Can you work these out from the model? Positions are in its coordinate system, mm. A direction names the side the tool comes from. Give positions to 0.01 mm unless a question says otherwise; leave off trailing zeros. Loops run counter-clockwise (first coordinate to the right, second up) from the corner with the lowest first, then second, coordinate; pieces in that order, holes last. Notation, with made-up numbers: (2.25, 85) - (32.25, 85) arc R8 ccw to (32.25, 91) - close; hole circle Ø4 at (65.25, 3). An arc over 180 degrees is marked (long way). Answer as a JSON object with one key per item and string values. Group by question number.
Item 1: Suppose I cut it at A-A on x = 0. Write out the boundary of the cut face in (y, z), and give its area (3 significant figures).
Item 2: Which directions (+Z, -Z, +X, -X, +Y, -Y) give clear straight access to the entire face, cutting with the end or side of a thin tool? Please do faces 4 (the flat face through (6, 0, -32.871)), 5 (the flat face through (-10, -10, -42.871)), 6 (the flat face through (6, 0, 32.871)), 7 (the conical face through (-40.938, 12.892, -29.206)), 8 (the cylindrical face through (49.45, 2.18, -38.84)).
Item 3: Please list where these lines run through material, in increasing order: L1, parallel to X at y = 0.5, z = 20.5; L2, parallel to Y at x = 0, z = 35; L3, parallel to Y at x = 0, z = 12.
Item 4: Suppose I cut it at C-C on z = 13. Write out the boundary of the cut face in (x, y).
Item 5: Thinking about a two-plate mould opening in Y: for faces 1 (the flat face through (10, -10, 42.871)), 2 (the cylindrical face through (9.21, -41.47, -0.4)), 3 (the cylindrical face through (-10.316, 7.91, -37.941)), which applies, pulls with the +Y half, pulls with the -Y half, needs draft (parallel to the pull), parting line crosses it, or undercut?
Item 6: Will these pins go through, and if not, where does the flat tip stop? pin 1 (12 mm diameter, centred on y = -29.5, z = -17.5, fed in from -X); pin 2 (8 mm diameter, centred on y = 22.5, z = -8.5, fed in from +X); pin 3 (5 mm diameter, centred on y = 16, z = -13.5, fed in from -X).
from build123d import *

# Parameters (mm, degrees)
F2_R     = 5
F3_DEPTH = 1000
F2_R_2   = 13
F4_DEPTH = 10
F5_R     = 13
F5_R_2   = 5
F6_DEPTH = 10


with BuildPart() as f1:
    # F0 (on Front) → F1 (revolve)
    with BuildSketch(Plane.XZ):
        Polygon((0, 0), (0, 42.870745), (-49.496219, 42.870745), (-49.496219, 34.686334), (-42.481005, 28.84032), (-42.481005, 0), (-42.481005, -28.84032), (-49.496219, -34.686334), (-49.496219, -42.870745), (0, -42.870745), align=None)
    revolve(axis=Axis((0, 0, 21.435373), (0, 0, -1)))

    # F2 (on face) → F3 (cut)
    with BuildSketch(Plane.XY.offset(42.870745)):
        Circle(F2_R)
    extrude(amount=-F3_DEPTH, mode=Mode.SUBTRACT)

    # F2 (on face) → F4 (cut)
    with BuildSketch(Plane.XY.offset(42.870745)):
        Circle(F2_R_2)
        Circle(F2_R, mode=Mode.SUBTRACT)
    extrude(amount=-F4_DEPTH, mode=Mode.SUBTRACT)

    # F5 (on face) → F6 (cut)
    with BuildSketch(Plane(origin=(0, 0, -42.870745), x_dir=(1, 0, 0), z_dir=(0, 0, -1))):
        Circle(F5_R)
        Circle(F5_R_2, mode=Mode.SUBTRACT)
    extrude(amount=-F6_DEPTH, mode=Mode.SUBTRACT)


solid = f1.part
Worked out:
{
 "1": {"outline": "(-49.5, -42.87) - (-13, -42.87) - (-13, -32.87) - (-5, -32.87) - (-5, 32.87) - (-13, 32.87) - (-13, 42.87) - (-49.5, 42.87) - (-49.5, 34.69) - (-42.48, 28.84) - (-42.48, -28.84) - (-49.5, -34.69) - close; (5, -32.87) - (13, -32.87) - (13, -42.87) - (49.5, -42.87) - (49.5, -34.69) - (42.48, -28.84) - (42.48, 28.84) - (49.5, 34.69) - (49.5, 42.87) - (13, 42.87) - (13, 32.87) - (5, 32.87) - close", "area": "6,420 mm2"},
 "2": {"face 4": "-Z", "face 5": "-Z, +X, -X, +Y, -Y", "face 6": "+Z", "face 7": "none", "face 8": "+Z, -Z"},
 "3": {"L1": "x = -42.48 to -4.97, 4.97 to 42.48", "L2": "y = -49.5 to -13, 13 to 49.5", "L3": "y = -42.48 to -5, 5 to 42.48"},
 "4": {"outline": "circle Ø84.96 at (0, 0); hole circle Ø10 at (0, 0)"},
 "5": {"face 1": "needs draft", "face 2": "parting line crosses it", "face 3": "undercut"},
 "6": {"pin 1": "stops at x = -35.39", "pin 2": "stops at x = 38.24", "pin 3": "stops at x = -40.28"}
}
